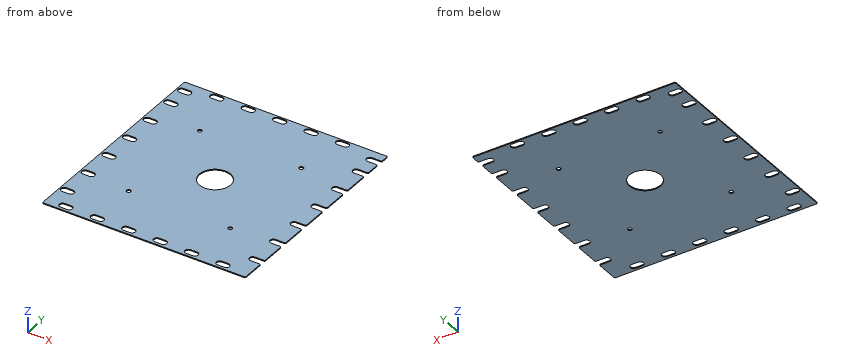
from build123d import *

# Parameters (mm, degrees)
SKETCH1_W               = 164.1
SKETCH1_H               = 174.745
SKETCH1_R               = 12.5
BOSS_EXTRUDE1_DEPTH     = 0.8
FILLET1_R               = 1
CUT_EXTRUDE1_DEPTH      = 241.06169004
CUT_EXTRUDE1_DEPTH_BACK = 241.06169004
SKETCH2_R               = 1.725
SKETCH2_W               = 2.675
SKETCH2_H               = 5.3
FILLET2_R               = 1


with BuildPart() as part:
    # Sketch1 → Boss-Extrude1 (new body)
    with BuildSketch(Plane.XY):
        with Locations((82.55, -87.3725)):
            Rectangle(SKETCH1_W, SKETCH1_H)
        with Locations((82.55, -87.3725)):
            Circle(SKETCH1_R, mode=Mode.SUBTRACT)
        with BuildLine():
            Line((82.55, -6.5), (77.25, -6.5))
            ThreePointArc((77.25, -6.5), (74.6, -3.85), (77.25, -1.2))
            Line((77.25, -1.2), (82.55, -1.2))
            ThreePointArc((82.55, -1.2), (85.2, -3.85), (82.55, -6.5))
        make_face(mode=Mode.SUBTRACT)
        with BuildLine():
            Line((13.75, -167.3325), (19.05, -167.3325))
            ThreePointArc((19.05, -167.3325), (21.7, -169.9825), (19.05, -172.6325))
            Line((19.05, -172.6325), (13.75, -172.6325))
            ThreePointArc((13.75, -172.6325), (11.1, -169.9825), (13.75, -167.3325))
        make_face(mode=Mode.SUBTRACT)
        with BuildLine():
            Line((4.225, -150.87), (9.525, -150.87))
            ThreePointArc((9.525, -150.87), (12.175, -153.52), (9.525, -156.17))
            Line((9.525, -156.17), (4.225, -156.17))
            ThreePointArc((4.225, -156.17), (1.575, -153.52), (4.225, -150.87))
        make_face(mode=Mode.SUBTRACT)
        with BuildLine():
            Line((39.15, -167.3325), (44.45, -167.3325))
            ThreePointArc((44.45, -167.3325), (47.1, -169.9825), (44.45, -172.6325))
            Line((44.45, -172.6325), (39.15, -172.6325))
            ThreePointArc((39.15, -172.6325), (36.5, -169.9825), (39.15, -167.3325))
        make_face(mode=Mode.SUBTRACT)
        with BuildLine():
            Line((64.55, -167.3325), (69.85, -167.3325))
            ThreePointArc((69.85, -167.3325), (72.5, -169.9825), (69.85, -172.6325))
            Line((69.85, -172.6325), (64.55, -172.6325))
            ThreePointArc((64.55, -172.6325), (61.9, -169.9825), (64.55, -167.3325))
        make_face(mode=Mode.SUBTRACT)
        with BuildLine():
            Line((4.225, -125.47), (9.525, -125.47))
            ThreePointArc((9.525, -125.47), (12.175, -128.12), (9.525, -130.77))
            Line((9.525, -130.77), (4.225, -130.77))
            ThreePointArc((4.225, -130.77), (1.575, -128.12), (4.225, -125.47))
        make_face(mode=Mode.SUBTRACT)
        with BuildLine():
            Line((4.225, -100.07), (9.525, -100.07))
            ThreePointArc((9.525, -100.07), (12.175, -102.72), (9.525, -105.37))
            Line((9.525, -105.37), (4.225, -105.37))
            ThreePointArc((4.225, -105.37), (1.575, -102.72), (4.225, -100.07))
        make_face(mode=Mode.SUBTRACT)
        with BuildLine():
            Line((4.225, -74.67), (9.525, -74.67))
            ThreePointArc((9.525, -74.67), (12.175, -77.32), (9.525, -79.97))
            Line((9.525, -79.97), (4.225, -79.97))
            ThreePointArc((4.225, -79.97), (1.575, -77.32), (4.225, -74.67))
        make_face(mode=Mode.SUBTRACT)
        with BuildLine():
            Line((4.225, -49.27), (9.525, -49.27))
            ThreePointArc((9.525, -49.27), (12.175, -51.92), (9.525, -54.57))
            Line((9.525, -54.57), (4.225, -54.57))
            ThreePointArc((4.225, -54.57), (1.575, -51.92), (4.225, -49.27))
        make_face(mode=Mode.SUBTRACT)
        with BuildLine():
            Line((4.225, -23.87), (9.525, -23.87))
            ThreePointArc((9.525, -23.87), (12.175, -26.52), (9.525, -29.17))
            Line((9.525, -29.17), (4.225, -29.17))
            ThreePointArc((4.225, -29.17), (1.575, -26.52), (4.225, -23.87))
        make_face(mode=Mode.SUBTRACT)
        with BuildLine():
            Line((4.225, -7.0375), (9.525, -7.0375))
            ThreePointArc((9.525, -7.0375), (12.175, -9.6875), (9.525, -12.3375))
            Line((9.525, -12.3375), (4.225, -12.3375))
            ThreePointArc((4.225, -12.3375), (1.575, -9.6875), (4.225, -7.0375))
        make_face(mode=Mode.SUBTRACT)
        with BuildLine():
            Line((26.45, -1.2), (31.75, -1.2))
            ThreePointArc((31.75, -1.2), (34.4, -3.85), (31.75, -6.5))
            Line((31.75, -6.5), (26.45, -6.5))
            ThreePointArc((26.45, -6.5), (23.8, -3.85), (26.45, -1.2))
        make_face(mode=Mode.SUBTRACT)
        with BuildLine():
            Line((51.85, -1.2), (57.15, -1.2))
            ThreePointArc((57.15, -1.2), (59.8, -3.85), (57.15, -6.5))
            Line((57.15, -6.5), (51.85, -6.5))
            ThreePointArc((51.85, -6.5), (49.2, -3.85), (51.85, -1.2))
        make_face(mode=Mode.SUBTRACT)
        with BuildLine():
            ThreePointArc((161.925, -7.0375), (164.575, -9.6875), (161.925, -12.3375))
            Line((161.925, -12.3375), (156.625, -12.3375))
            ThreePointArc((156.625, -12.3375), (153.975, -9.6875), (156.625, -7.0375))
            Line((156.625, -7.0375), (161.925, -7.0375))
        make_face(mode=Mode.SUBTRACT)
        with BuildLine():
            Line((89.95, -167.3325), (95.25, -167.3325))
            ThreePointArc((95.25, -167.3325), (97.9, -169.9825), (95.25, -172.6325))
            Line((95.25, -172.6325), (89.95, -172.6325))
            ThreePointArc((89.95, -172.6325), (87.3, -169.9825), (89.95, -167.3325))
        make_face(mode=Mode.SUBTRACT)
        with BuildLine():
            Line((115.35, -167.3325), (120.65, -167.3325))
            ThreePointArc((120.65, -167.3325), (123.3, -169.9825), (120.65, -172.6325))
            Line((120.65, -172.6325), (115.35, -172.6325))
            ThreePointArc((115.35, -172.6325), (112.7, -169.9825), (115.35, -167.3325))
        make_face(mode=Mode.SUBTRACT)
        with BuildLine():
            Line((140.75, -167.3325), (146.05, -167.3325))
            ThreePointArc((146.05, -167.3325), (148.7, -169.9825), (146.05, -172.6325))
            Line((146.05, -172.6325), (140.75, -172.6325))
            ThreePointArc((140.75, -172.6325), (138.1, -169.9825), (140.75, -167.3325))
        make_face(mode=Mode.SUBTRACT)
        with BuildLine():
            Line((156.625, -150.87), (161.925, -150.87))
            ThreePointArc((161.925, -150.87), (164.575, -153.52), (161.925, -156.17))
            Line((161.925, -156.17), (156.625, -156.17))
            ThreePointArc((156.625, -156.17), (153.975, -153.52), (156.625, -150.87))
        make_face(mode=Mode.SUBTRACT)
        with BuildLine():
            Line((156.625, -125.47), (161.925, -125.47))
            ThreePointArc((161.925, -125.47), (164.575, -128.12), (161.925, -130.77))
            Line((161.925, -130.77), (156.625, -130.77))
            ThreePointArc((156.625, -130.77), (153.975, -128.12), (156.625, -125.47))
        make_face(mode=Mode.SUBTRACT)
        with BuildLine():
            Line((156.625, -100.07), (161.925, -100.07))
            ThreePointArc((161.925, -100.07), (164.575, -102.72), (161.925, -105.37))
            Line((161.925, -105.37), (156.625, -105.37))
            ThreePointArc((156.625, -105.37), (153.975, -102.72), (156.625, -100.07))
        make_face(mode=Mode.SUBTRACT)
        with BuildLine():
            Line((156.625, -74.67), (161.925, -74.67))
            ThreePointArc((161.925, -74.67), (164.575, -77.32), (161.925, -79.97))
            Line((161.925, -79.97), (156.625, -79.97))
            ThreePointArc((156.625, -79.97), (153.975, -77.32), (156.625, -74.67))
        make_face(mode=Mode.SUBTRACT)
        with BuildLine():
            Line((156.625, -49.27), (161.925, -49.27))
            ThreePointArc((161.925, -49.27), (164.575, -51.92), (161.925, -54.57))
            Line((161.925, -54.57), (156.625, -54.57))
            ThreePointArc((156.625, -54.57), (153.975, -51.92), (156.625, -49.27))
        make_face(mode=Mode.SUBTRACT)
        with BuildLine():
            Line((102.65, -1.2), (107.95, -1.2))
            ThreePointArc((107.95, -1.2), (110.6, -3.85), (107.95, -6.5))
            Line((107.95, -6.5), (102.65, -6.5))
            ThreePointArc((102.65, -6.5), (100, -3.85), (102.65, -1.2))
        make_face(mode=Mode.SUBTRACT)
        with BuildLine():
            Line((156.625, -23.87), (161.925, -23.87))
            ThreePointArc((161.925, -23.87), (164.575, -26.52), (161.925, -29.17))
            Line((161.925, -29.17), (156.625, -29.17))
            ThreePointArc((156.625, -29.17), (153.975, -26.52), (156.625, -23.87))
        make_face(mode=Mode.SUBTRACT)
        with BuildLine():
            Line((128.05, -1.2), (133.35, -1.2))
            ThreePointArc((133.35, -1.2), (136, -3.85), (133.35, -6.5))
            Line((133.35, -6.5), (128.05, -6.5))
            ThreePointArc((128.05, -6.5), (125.4, -3.85), (128.05, -1.2))
        make_face(mode=Mode.SUBTRACT)
    extrude(amount=BOSS_EXTRUDE1_DEPTH)

    # Fillet1
    fillet1_edges = [part.edges().sort_by_distance(p)[0] for p in [
        (0.5, -174.745, 0.4),
        (0.5, 0, 0.4),
        (164.6, 0, 0.4),
        (164.6, -174.745, 0.4),
    ]]
    fillet(fillet1_edges, radius=FILLET1_R)

    # Sketch2 → Cut-Extrude1 (cut, two sides: drawn at the far end of the back side and taken through both)
    with BuildSketch(Plane.XY.offset(0.8).offset(-CUT_EXTRUDE1_DEPTH_BACK)):
        with Locations((41.525, -43.68625)):
            Circle(SKETCH2_R)
        with Locations((123.575, -43.68625)):
            Circle(SKETCH2_R)
        with Locations((123.575, -131.05875)):
            Circle(SKETCH2_R)
        with Locations((41.525, -131.05875)):
            Circle(SKETCH2_R)
        with Locations((163.2625, -9.6875)):
            Rectangle(SKETCH2_W, SKETCH2_H)
        with Locations((163.2625, -51.92)):
            Rectangle(SKETCH2_W, SKETCH2_H)
        with Locations((163.2625, -26.52)):
            Rectangle(SKETCH2_W, SKETCH2_H)
        with Locations((163.2625, -77.32)):
            Rectangle(SKETCH2_W, SKETCH2_H)
        with Locations((163.2625, -102.72)):
            Rectangle(SKETCH2_W, SKETCH2_H)
        with Locations((163.2625, -128.12)):
            Rectangle(SKETCH2_W, SKETCH2_H)
        with Locations((163.2625, -153.52)):
            Rectangle(SKETCH2_W, SKETCH2_H)
    extrude(amount=CUT_EXTRUDE1_DEPTH + CUT_EXTRUDE1_DEPTH_BACK, mode=Mode.SUBTRACT)

    # Fillet2
    fillet2_edges = [part.edges().sort_by_distance(p)[0] for p in [
        (164.6, -100.07, 0.4),
        (164.6, -105.37, 0.4),
        (164.6, -74.67, 0.4),
        (164.6, -79.97, 0.4),
        (164.6, -49.27, 0.4),
        (164.6, -54.57, 0.4),
        (164.6, -23.87, 0.4),
        (164.6, -29.17, 0.4),
        (164.6, -7.0375, 0.4),
        (164.6, -12.3375, 0.4),
        (164.6, -125.47, 0.4),
        (164.6, -130.77, 0.4),
        (164.6, -150.87, 0.4),
        (164.6, -156.17, 0.4),
    ]]
    fillet(fillet2_edges, radius=FILLET2_R)


solid = part.part
Part model, mm, in its own coordinate system. Coordinates: 2 decimals unless noted, no trailing zeros. Loops run counter-clockwise (first coordinate to the right, second up) from the corner with the lowest first, then second, coordinate; pieces in that order, holes last. Notation, with made-up numbers: (20.5, -37.5) -> (41.5, -37.5) arc R20 cw to (41.5, -11.5) -> close; hole circle Ø2 at (34.25, 85). An arc over 180 degrees is marked (long way). Use a Markdown table: item, result. Add a question column.
Item 1: Probe probe 1 along Y at (x, z) = (82.55, 0.25) (1 decimal); probe 2 along Y at (x, z) = (57, 0.45) (3 decimals); probe 3 along Y at (x, z) = (119, 0.4) (1 decimal). List the from-to ranges inside material, lowest first.
Item 2: Flat gauge pin, fed straight in: P1, Ø22.5, axis at x = 82.55, y = -87.37, coming from the -Z side. Where does the tip first touch, or does it go through?
Item 3: Band-saw the part on B-B on y = -78. Write the cut outline in (x, z).
Item 4: Band-saw the part on C-C on z = 0.55. Give the number of separate pieces and of enclosed holes in the cut face, plus the area to 3 significant figures.
Item 5: Band-saw the part on A-A on y = -51.92. Write the cut outline in (x, z) (3 decimals), plus the area to 3 significant figures.
Geometry says:
| question | item | result |
|---|---|---|
| 1 | probe 1 | -174.7 to -99.9, -74.9 to -6.5, -1.2 to 0 |
| 1 | probe 2 | -174.745 to -6.5, -1.2 to 0 |
| 1 | probe 3 | -174.7 to -172.6, -167.3 to 0 |
| 2 | P1 | through |
| 3 | outline | (0.5, 0) -> (1.66, 0) -> (1.66, 0.8) -> (0.5, 0.8) -> close; (12.09, 0) -> (74.28, 0) -> (74.28, 0.8) -> (12.09, 0.8) -> close; (90.82, 0) -> (154.06, 0) -> (154.06, 0.8) -> (90.82, 0.8) -> close |
| 4 | separate pieces | 1 |
| 4 | enclosed holes | 23 |
| 4 | area | 26,900 mm² |
| 5 | outline | (0.5, 0) -> (1.575, 0) -> (1.575, 0.8) -> (0.5, 0.8) -> close; (12.175, 0) -> (153.975, 0) -> (153.975, 0.8) -> (12.175, 0.8) -> close |
| 5 | area | 114 mm² |
